Geometry: final body of the model. Coordinates: model frame, mm. Face numbers are marked on the shaded views. A direction names the side the tool comes from. Give positions to 0.01 mm unless a question says otherwise; leave off trailing zeros. Write each loop counter-clockwise with the first axis right and the second up, starting at its lowest first coordinate (ties: lowest second). Pieces come first, ordered by that corner, then holes. Notation, with made-up numbers: M 6,-33.75 L 23,-33.75 A18 cw 23,-21.75 Z; hole C -7,46.5 d2. An arc over 180 degrees is marked long. Use a Markdown table: item, result. Add a question column.
(1) Cut plane C-C (x = 207.5). Output: boundary loops of the cut face in (y, z), plus the area to 3 significant figures.
(2) Reachability of the marked faces 1 and 2 from +Z, -Z, +X, -X, +Y, -Y: full face, straight path, thin tool, end or side. Return the list, or none.
(3) Draft query along Y for the marked faces 3 and 4. Return one class per face: released by +Y, released by -Y, zero draft, split by the parting line, or undercut.
(4) Material intervals for L1, parallel to X at y = -558.5, z = 969.5; L2, parallel to Z at x = 140.5, y = -407; L3, parallel to Z at x = 513, y = -74, sorted ascending.
(5) Cut plane B-B (y = -431). Output: boundary loops of the cut face in (x, z), plus the area to 3 significant figures.
(6) Cut plane A-A (z = 426.5). Output: boundary loops of the cut face in (x, y), plus the area to 3 significant figures.
(7) Pin query (flat end, axial travel): pin 1 Ø10 at (x, y) = (939.5, -1074.5) entering from -Z. Return the tip coordinate at first contact, or that it passes through.
```python
from build123d import *

# Parameters (mm, degrees)
F1_DEPTH = 1800
F2_W     = 76
F2_H     = 76
F3_DEPTH = 1300


with BuildPart() as f1:
    # F0 (on Front) → F1 (new body)
    with BuildSketch(Plane.XZ):
        Polygon((2.1745097741, -49.5584370656), (2.1745097741, 1446.4415629344), (-1.8254902259, 1446.4415629344), (-1.8254902259, -53.5584370656), (1298.1745097741, -53.5584370656), (1298.1745097741, 1446.4415629344), (1294.1745097741, 1446.4415629344), (1294.1745097741, -49.5584370656), align=None)
    extrude(amount=F1_DEPTH)

    # F2 (on face) → F3 (join)
    with BuildSketch(Plane.YZ.offset(1298.1745097741)):
        with Locations((-38, -91.5584370656)):
            Rectangle(F2_W, F2_H)
        with Locations((-1762, -91.5584370656)):
            Rectangle(F2_W, F2_H)
    extrude(amount=-F3_DEPTH)


solid = f1.part
```
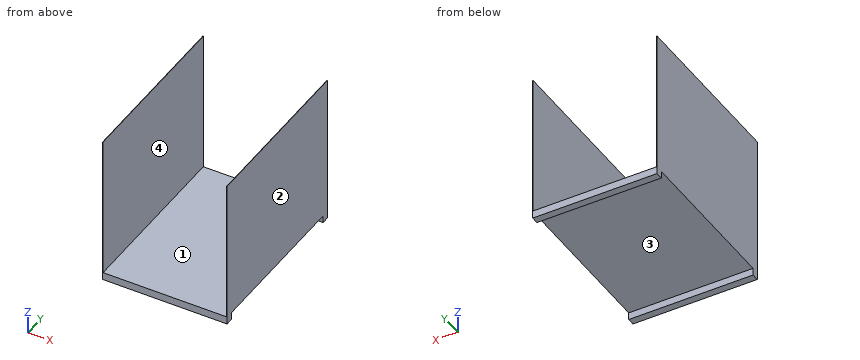
Answer list:
| question | item | result |
|---|---|---|
| 1 | outline | M -1800,-129.56 L -1724,-129.56 L -1724,-53.56 L -76,-53.56 L -76,-129.56 L 0,-129.56 L 0,-49.56 L -1800,-49.56 Z |
| 1 | area | 18,800 mm² |
| 2 | face 1 | +Z, +Y, -Y |
| 2 | face 2 | +Z, -Z, +X, +Y, -Y |
| 3 | face 3 | undercut |
| 3 | face 4 | zero draft |
| 4 | L1 | -1.83 to 2.17, 1294.17 to 1298.17 |
| 4 | L2 | -53.56 to -49.56 |
| 4 | L3 | -129.56 to -49.56 |
| 5 | outline | M -1.83,-53.56 L 1298.17,-53.56 L 1298.17,1446.44 L 1294.17,1446.44 L 1294.17,-49.56 L 2.17,-49.56 L 2.17,1446.44 L -1.83,1446.44 Z |
| 5 | area | 17,200 mm² |
| 6 | outline | M -1.83,-1800 L 2.17,-1800 L 2.17,0 L -1.83,0 Z; M 1294.17,-1800 L 1298.17,-1800 L 1298.17,0 L 1294.17,0 Z |
| 6 | area | 14,400 mm² |
| 7 | pin 1 | z = -53.56 |
